Can you work these out from the model? Positions are in its coordinate system, mm. Face numbers are marked on the shaded views. A direction names the side the tool comes from. Coordinates: 2 decimals unless noted, no trailing zeros. Order: outer loops, then holes, each group sorted by start corner. A loop starts at its lowest first (then second) coordinate and runs counter-clockwise, first axis right, second up. Notation, with made-up numbers: (-18, 48.25) -> (14, 48.25) arc R23 cw to (14, 76.25) -> close; hole circle Ø10 at (34, 18.5). An arc over 180 degrees is marked (long way). Answer in a Markdown table with one row per item. Add a question column.
1. On a 3-axis mill with a long thin cutter (end or side, diameter ignored), from which of +Z, -Z, +X, -X, +Y, -Y can I reach the whole of each face in a straight line? I mean the marked faces 1, 2 and 3. Say none if no direction works.
2. Imagine slicing it at C-C on y = 7.25. Write out the boundary of the cut face in (x, z), plus the area to 3 significant figures.
3. Imagine slicing it at D-D on z = 0.3. Write out the boundary of the cut face in (x, y) (3 decimals), plus the area to 3 significant figures.
4. Will these pins go through, and if not, where does the flat tip stop? pin 1 (1.8 mm diameter, centred on x = 4, y = -2, fed in from +Z); pin 2 (1.6 mm diameter, centred on x = 2, y = 1, fed in from +Z); pin 3 (2.5 mm diameter, centred on x = 0, y = -6.985, fed in from +Z).
5. We'd pull the mould along X, two halves only. Please class the marked faces 4, 5 and 6: pulls with the +X half, pulls with the -X half, needs draft (parallel to the pull), parting line crosses it, or undercut.
6. If I drill on line 1 along Y through (x, z) = (0, 0.5) (3 decimals); line 2 along Y through (x, z) = (-0.5, 2.3) (3 decimals); line 3 along Y through (x, z) = (1, 1.15) (3 decimals), over which ranges is the centre line in solid material (lowest first)? Write a range as [from, to].
7. Imagine slicing it at B-B on y = -1.25. Write out the boundary of the cut face in (x, z), plus the area to 3 significant figures.
8. Imagine slicing it at A-A on x = 0. State how many separate pieces and enclosed holes the cut face has, plus the area to 3 significant figures.
from build123d import *

# Parameters (mm, degrees)
SKETCH1_W           = 12.7
SKETCH1_H           = 19.05
SKETCH1_R           = 1.65
BOSS_EXTRUDE1_DEPTH = 1.5875
SKETCH2_W           = 12.7
SKETCH2_H           = 5.55625
SKETCH2_R           = 1.65
BOSS_EXTRUDE2_DEPTH = 0.889
BOSS_EXTRUDE3_REACH = 17.117
LPATTERN1_COUNT     = 2
LPATTERN1_PITCH     = 4.318
LPATTERN1_COL_COUNT = 2
LPATTERN1_COL_PITCH = 4.318


with BuildPart() as part:
    # Sketch1 → Boss-Extrude1 (new body)
    with BuildSketch(Plane.XY):
        Rectangle(SKETCH1_W, SKETCH1_H)
        with Locations((0, 6.985)):
            Circle(SKETCH1_R, mode=Mode.SUBTRACT)
        with Locations(Location((0, -6.985, 0), (0, 0, 180))):
            Circle(SKETCH1_R, mode=Mode.SUBTRACT)
    extrude(amount=BOSS_EXTRUDE1_DEPTH)

    # Sketch2 → Boss-Extrude2 (add)
    # profile 1 of 2: a face of its own
    with BuildSketch(Plane.XY.offset(1.5875)):
        with Locations((0, -6.746875)):
            Rectangle(SKETCH2_W, SKETCH2_H)
        with Locations(Location((0, -6.985, 0), (0, 0, 180))):
            Circle(SKETCH2_R, mode=Mode.SUBTRACT)
    # profile 2 of 2: a face of its own
    with BuildSketch(Plane.XY.offset(1.5875)):
        with Locations((0, 6.746875)):
            Rectangle(SKETCH2_W, SKETCH2_H)
        with Locations((0, 6.985)):
            Circle(SKETCH2_R, mode=Mode.SUBTRACT)
    extrude(amount=BOSS_EXTRUDE2_DEPTH)

    # Sketch3 → Boss-Extrude3 (add, up to next)
    with BuildSketch(Plane.XZ.offset(-3.96875), mode=Mode.PRIVATE) as boss_extrude3_sk1:
        with BuildLine():
            Line((-0.8001, 2.0955), (0.8001, 2.0955))
            ThreePointArc((0.8001, 2.0955), (0.873917251, 2.071844151), (0.920235135, 2.009689189))
            Line((0.920235135, 2.009689189), (1.035564865, 1.673310811))
            ThreePointArc((1.035564865, 1.673310811), (1.081882749, 1.611155849), (1.1557, 1.5875))
            Line((1.1557, 1.5875), (-1.1557, 1.5875))
            ThreePointArc((-1.1557, 1.5875), (-1.081882749, 1.611155849), (-1.035564865, 1.673310811))
            Line((-1.035564865, 1.673310811), (-0.920235135, 2.009689189))
            ThreePointArc((-0.920235135, 2.009689189), (-0.873917251, 2.071844151), (-0.8001, 2.0955))
        make_face()
    boss_extrude3_tool1 = extrude(boss_extrude3_sk1.sketch, amount=BOSS_EXTRUDE3_REACH, mode=Mode.PRIVATE) - part.part
    boss_extrude3 = boss_extrude3_tool1.solids().sort_by_distance((0, 3.96875, 1.832521))[0]
    add(boss_extrude3)

    # LPattern1: Boss-Extrude3 ×2
    with Locations(*[(i * LPATTERN1_PITCH, 0, 0) for i in range(1, LPATTERN1_COUNT)]):
        add(boss_extrude3)

    # LPattern1 col: Boss-Extrude3 ×2
    with Locations(*[(-i * LPATTERN1_COL_PITCH, 0, 0) for i in range(1, LPATTERN1_COL_COUNT)]):
        add(boss_extrude3)


solid = part.part
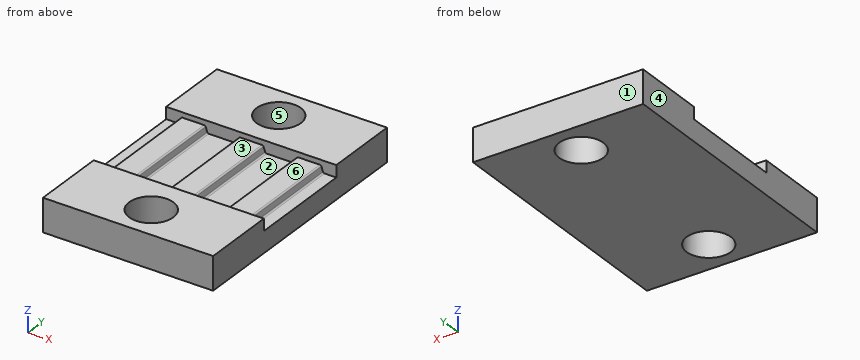
Answers follow:
| question | item | result |
|---|---|---|
| 1 | face 1 | +Z, -Z, +X, -X, +Y |
| 1 | face 2 | +Z |
| 1 | face 3 | +Z, +X, -X |
| 2 | outline | (-6.35, 0) -> (-1.63, 0) -> (-1.63, 2.48) -> (-6.35, 2.48) -> close; (1.63, 0) -> (6.35, 0) -> (6.35, 2.48) -> (1.63, 2.48) -> close |
| 2 | area | 23.4 mm² |
| 3 | outline | (-6.35, -9.525) -> (6.35, -9.525) -> (6.35, 9.525) -> (-6.35, 9.525) -> close; hole circle Ø3.3 at (0, -6.985); hole circle Ø3.3 at (0, 6.985) |
| 3 | area | 225 mm² |
| 4 | pin 1 | stops at z = 2.1 |
| 4 | pin 2 | stops at z = 1.59 |
| 4 | pin 3 | passes through |
| 5 | face 4 | pulls with the -X half |
| 5 | face 5 | undercut |
| 5 | face 6 | needs draft |
| 6 | line 1 | y = [-9.525, -8.635], [-5.335, 5.335], [8.635, 9.525] |
| 6 | line 2 | y = [-9.525, -8.557], [-5.413, -3.969], [3.969, 5.413], [8.557, 9.525] |
| 6 | line 3 | y = [-9.525, -8.297], [-5.673, 5.673], [8.297, 9.525] |
| 7 | outline | (-6.35, 0) -> (6.35, 0) -> (6.35, 1.59) -> (5.47, 1.59) arc R0.13 cw to (5.35, 1.67) -> (5.24, 2.01) arc R0.13 ccw to (5.12, 2.1) -> (3.52, 2.1) arc R0.13 ccw to (3.4, 2.01) -> (3.28, 1.67) arc R0.13 cw to (3.16, 1.59) -> (1.16, 1.59) arc R0.13 cw to (1.04, 1.67) -> (0.92, 2.01) arc R0.13 ccw to (0.8, 2.1) -> (-0.8, 2.1) arc R0.13 ccw to (-0.92, 2.01) -> (-1.04, 1.67) arc R0.13 cw to (-1.16, 1.59) -> (-3.16, 1.59) arc R0.13 cw to (-3.28, 1.67) -> (-3.4, 2.01) arc R0.13 ccw to (-3.52, 2.1) -> (-5.12, 2.1) arc R0.13 ccw to (-5.24, 2.01) -> (-5.35, 1.67) arc R0.13 cw to (-5.47, 1.59) -> (-6.35, 1.59) -> close |
| 7 | area | 23.1 mm² |
| 8 | separate pieces | 3 |
| 8 | enclosed holes | 0 |
| 8 | area | 27.8 mm² |
